```python
from build123d import *

# Parameters (mm, degrees)
F0_R     = 3.725
F1_DEPTH = 1.5
F2_R     = 1.725
F3_DEPTH = 3.5
F4_R     = 1.725
F5_DEPTH = 1.6
F6_SIZE  = 0.6


with BuildPart() as f1:
    # F0 (on Right) → F1 (new body)
    with BuildSketch(Plane.YZ):
        Circle(F0_R)
    extrude(amount=F1_DEPTH)

    # F2 (on Right) → F3 (join)
    with BuildSketch(Plane.YZ):
        Circle(F2_R)
    extrude(amount=-F3_DEPTH)

    # F4 (on Right) → F5 (join)
    with BuildSketch(Plane.YZ):
        Circle(F4_R)
    extrude(amount=F5_DEPTH)

    # F6
    f6_edges = [f1.edges().sort_by_distance(p)[0] for p in [
        (-3.5, -1.725, 0),
    ]]
    chamfer(f6_edges, length=F6_SIZE)


solid = f1.part
```
Source: CAD feature listing. Evaluate the final solid. Frame: model axes, mm. A direction names the side the tool comes from. Round coordinates to 2 decimals unless told otherwise and drop trailing zeros. Loops run counter-clockwise (first coordinate to the right, second up) from the corner with the lowest first, then second, coordinate; pieces in that order, holes last.
(1) Material intervals for probe 1 along X at (y, z) = (2.25, 0.75); probe 2 along Z at (x, y) = (-1.2, 0) (3 decimals); probe 3 along Z at (x, y) = (1.3, -1.25), sorted ascending.
From the geometry:
probe 1: x = 0 to 1.5
probe 2: z = -1.725 to 1.725
probe 3: z = -3.51 to 3.51
(2) Section query A-A (z = 0). Output: boundary loops of the cut face in (x, y) (3 decimals).
From the geometry:
outline: (-3.5, -1.125) - (-2.9, -1.725) - (0, -1.725) - (0, -3.725) - (1.5, -3.725) - (1.5, -1.725) - (1.6, -1.725) - (1.6, 1.725) - (1.5, 1.725) - (1.5, 3.725) - (0, 3.725) - (0, 1.725) - (-2.9, 1.725) - (-3.5, 1.125) - close
(3) Access query for faces 1 (the flat face through (1.6, 0, 0)), 2 (the flat face through (0, 1, -2)), 3 (the flat face through (1.5, 1, -2)). Directions: +Z, -Z, +X, -X, +Y, -Y. A direction counts if a zero-diameter tool reaches every point of the face in a straight line with its end or side. Return the directions, or none.
From the geometry:
face 1: +Z, -Z, +X, +Y, -Y
face 2: -X
face 3: +X
(4) Section query C-C (x = -2.6). Output: boundary loops of the cut face in (y, z) (3 decimals), and give its area (3 significant figures).
From the geometry:
outline: circle Ø3.45 at (0, 0)
area: 9.35 mm2
(5) Contact query for flat-ended pins moving along their axis: pin 1 Ø1 at (x, y) = (0.5, -1.5) entering from +Z; pin 2 Ø3 at (y, z) = (2.5, -2.5) entering from -X. Output: stop coordinate, or through.
From the geometry:
pin 1: stops at z = 3.59
pin 2: stops at x = 0
(6) Section query D-D (y = -3). Output: boundary loops of the cut face in (x, z), and give its area (3 significant figures).
From the geometry:
outline: (0, -2.21) - (1.5, -2.21) - (1.5, 2.21) - (0, 2.21) - close
area: 6.62 mm2
